Autodesk Inventor part; units mm, degrees
ref_plane "Arbeitsebene1" through (100.3058, 53.4709, 0) normal (0, -1, 0) x (1, 0, 0)
ref_plane "YZ Plane" through (0, 0, 0) normal (1, 0, 0) x (0, 1, 0)
ref_plane "XZ Plane" through (0, 0, 0) normal (0, 1, 0) x (-1, 0, 0)
sketch "Skizze1" plane through (0, 0, 0) normal (0, 0, 1) x (1, 0, 0)
  line L0 (0, 0) -> (0, 15)
  arc A0 (150, 45) -> (0, 15) centre (100.3058, -96.5291) ccw
  line L1 (150, 45) -> (150, -15)
  line L2 (150, -15) -> (120, -15)
  arc A1 (120, -15) -> (0, 0) centre (41.6262, -154.4903) ccw
  dimension "hoehe2" = 60
  dimension "Durchmesser" = 160
  dimension "Durchmesser2" = 150
  dimension "Breite1" = 30
  dimension "d12" = 120
  dimension "Höhe1" = 15
  dimension "d14" = 15
extrude "Extrusion1" add sketch "Skizze1" along normal blind 60
ref_plane "Arbeitsebene1" through (100.3058, 53.4709, 0) normal (0, -1, 0) x (1, 0, 0)
sketch "Skizze2" plane through (100.3058, 53.4709, 0) normal (0, -1, 0) x (1, 0, 0)
  line L0 (-100.3058, 0) -> (-100.3058, 60)
  line L1 (-100.3058, 51.4359) -> (-20.3058, 30)
  line L2 (-20.3058, 30) -> (-100.3058, 8.5641)
  line L3 (-100.3058, 30) -> (-9.7877, 30) construction
  dimension "d17" = 30
  dimension "d18" = 80
extrude "Extrusion2" cut sketch "Skizze2" along normal up to surface
sketch "Skizze3" plane through (150, -15, 0) normal (1, 0, 0) x (0, 0, -1)
  circle A0 centre (-30, 30) radius 15
  line L0 (0, 0) -> (0, 60)
  line L1 (0, 0) -> (-60, 0)
  point P0 (0, 15)
  point P1 (0, 30)
  point P2 (-30, 0)
  dimension "d21" = 30
extrude "Extrusion3" add sketch "Skizze3" along normal blind 20
sketch "Skizze4" plane through (170, 15, 30) normal (1, 0, 0) x (0, 0, -1)
  line L0 (0, 37.0901) -> (0, -14.1602)
  circle A0 centre (0, 0) radius 25
  line L1 (30, -30) -> (30, 30)
  point P0 (30, -15)
  point P1 (30, 0)
  dimension "d24" = 50
extrude "Extrusion4" add sketch "Skizze4" along normal blind 20
fillet "Rundung1" radius 5 1 edges at (190, 15, 55)
properties part number "practice3" material "Phenolharz"
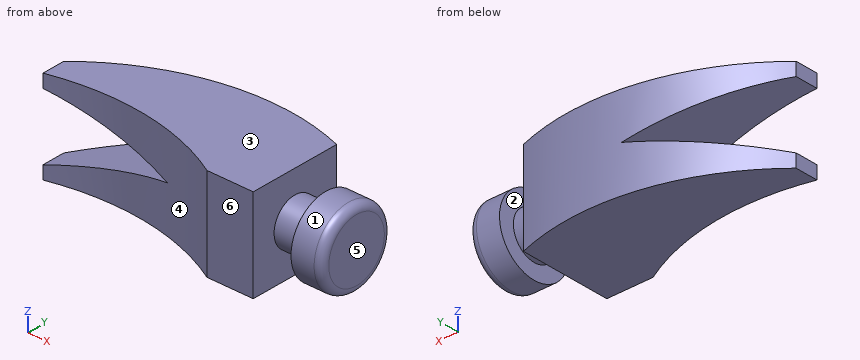
Part model, mm, in its own coordinate system. Face numbers are marked on the shaded views. A direction names the side the tool comes from. Round coordinates to 2 decimals unless told otherwise and drop trailing zeros. Order: outer loops, then holes, each group sorted by start corner. A loop starts at its lowest first (then second) coordinate and runs counter-clockwise, first axis right, second up. Notation, with made-up numbers: M -12,44 L 37,44 A26 cw 37,74 Z; hole C 13,61 d6. An arc over 180 degrees is marked long. Put each result on its own line as item: value. Start each with the question number.
1. Drill centre lines: probe 1 along Y at (x, z) = (158, 31); probe 2 along X at (y, z) = (13.5, 4.5); probe 3 along Z at (x, y) = (44, 31). Where is each one in solid material? Low to high. Write a range as [from, to].
2. Tool access for the marked faces 1, 2 and 3: list every direction of +Z, -Z, +X, -X, +Y, -Y with a clear straight run to the whole face (end or side of a thin tool).
3. Slice it at A-A on x = 43.5. List the corners of the cut face in (y, z).
4. Slice it at B-B on x = 176. List the corners of the cut face in (y, z).
5. Two-plate mould, pull along X, no slides. Class the marked faces 4, 5 and 6: +X half, -X half, draft (parallel to the pull), parting line (faces both ways), or undercut.
6. Drop flat-ended pins along their axis: pin 1 (4 mm diameter, centred on x = 126, z = 46.5, fed in from +Y); pin 2 (8 mm diameter, centred on x = 165, z = 25, fed in from +Y); pin 3 (10 mm diameter, centred on x = 36.5, z = 12, fed in from -Y). Give the stop position or say it passes through.
Findings:
1. probe 1: [0.03, 29.97]
1. probe 2: [0, 150]
1. probe 3: [0, 20.35], [39.65, 60]
2. face 1: +X
2. face 2: none
2. face 3: +Z, +X, -X, +Y, -Y
3. outline: M 5.5,0 L 42.3,0 L 42.3,20.22 L 5.5,20.22 Z; M 5.5,39.78 L 42.3,39.78 L 42.3,60 L 5.5,60 Z
4. outline: C 15,30 d50
5. face 4: undercut
5. face 5: +X half
5. face 6: draft
6. pin 1: y = 51.59
6. pin 2: y = 29.97
6. pin 3: y = 5.19
